Source: CAD feature listing. Evaluate the final solid. Frame: model axes, mm. A direction names the side the tool comes from. Give positions to 0.01 mm unless a question says otherwise; leave off trailing zeros. Write each loop counter-clockwise with the first axis right and the second up, starting at its lowest first coordinate (ties: lowest second). Pieces come first, ordered by that corner, then holes. Notation, with made-up numbers: (56.25, 19) - (61.25, 19) arc R11 cw to (61.25, 34) - close; hole circle Ø3 at (2.25, -19.75). An arc over 180 degrees is marked (long way). One line per question, with ' | ' between items. Start each with the question number.
(1) Section C-C, the plane x = -19.5. Return loops of the section in (y, z), plus the area to 3 significant figures.
(2) Draft query along Z for faces 4 (the flat face through (2.1, 0.7, -9)), 5 (the flat face through (-25.3, 5, -13.7)), 6 (the cylindrical face through (-26.58, 1.23, -17.6)), 7 (the cylindrical face through (26.58, 1.23, 17.6)). Return one class per face: +Z half, -Z half, draft (parallel to the pull), parting line (faces both ways), or undercut.
(3) Pin query (flat end, axial travel): pin 1 (1.9 mm diameter, centred on x = -24, z = 15, fed in from -Y); pin 2 (8 mm diameter, centred on x = -19, z = 6, fed in from +Y); pin 3 (1.7 mm diameter, centred on x = -0.5, z = 13, fed in from +Y). Return the tip coordinate at first contact, or that it passes through.
(4) Section B-B, the plane z = -7. Return loops of the section in (x, y), plus the area to 3 significant figures.
(5) Access query for faces 1 (the flat face through (4, 1, 0)), 2 (the flat face through (22.7, 5, -13.7)), 3 (the cylindrical face through (-24, 4, -18)). Directions: +Z, -Z, +X, -X, +Y, -Y. A direction counts if a zero-diameter tool reaches every point of the face in a straight line with its end or side. Return the directions, or none.
(6) Section A-A, the plane y = 4.1. Return loops of the section in (x, z), plus the area to 3 significant figures.
(7) Ray query, line 1 (Z direction, x = 24, y = 1.6); line 2 (X direction, y = 1.9, z = 15); line 3 (Z direction, x = -3, y = 2). Return the intervals inside material, ascending. Write a range as [from, to].
```python
from build123d import *

# Parameters (mm, degrees)
SKETCH_1_R           = 1.55
EXTRUDE_1_DEPTH      = 2.5
SKETCH_2_R           = 3
EXTRUDE_2_DEPTH      = 2.5
SKETCH_3_R           = 1.55
CUT_EXTRUDE_1_DEPTH  = 34.466573357
SKETCH_5_R           = 3.5
CUT_EXTRUDE_3_DEPTH  = 34.466573357
CUT_EXTRUDE_6_DEPTH  = 1.5
FILLET_4_R           = 0.5
CHAMFER_1_SIZE       = 2
CHAMFER_1_SIZE2      = 1
FILLET_5_R           = 1
CUT_EXTRUDE_7_DEPTH  = 34.466573357
SKETCH_20_W          = 5
SKETCH_20_H          = 18
CUT_EXTRUDE_10_DEPTH = 34.486179612
FILLET_9_R           = 1
SKETCH_23_R          = 1.05
CUT_EXTRUDE_11_DEPTH = 34.466573357
FILLET_10_R          = 1


with BuildPart() as part:
    # Sketch 1 → Extrude 1 (new body)
    with BuildSketch(Plane(origin=(0, 0, 0), x_dir=(1, 0, 0), z_dir=(0, 1, 0))):
        with BuildLine():
            Line((-27.4365, 0), (-27.4365, 15.5))
            ThreePointArc((-27.4365, 15.5), (-26.557820344, 17.621320344), (-24.4365, 18.5))
            Line((-24.4365, 18.5), (0, 18.5))
            Line((0, 18.5), (24.4365, 18.5))
            ThreePointArc((24.4365, 18.5), (26.557820344, 17.621320344), (27.4365, 15.5))
            Line((27.4365, 15.5), (27.4365, 0))
            Line((27.4365, 0), (27.4365, -15.5))
            ThreePointArc((27.4365, -15.5), (26.557820344, -17.621320344), (24.4365, -18.5))
            Line((24.4365, -18.5), (0, -18.5))
            Line((0, -18.5), (-24.4365, -18.5))
            ThreePointArc((-24.4365, -18.5), (-26.557820344, -17.621320344), (-27.4365, -15.5))
            Line((-27.4365, -15.5), (-27.4365, 0))
        make_face()
        with Locations(Location((-24, 15, 0), (0, 0, 270))):
            Circle(SKETCH_1_R, mode=Mode.SUBTRACT)
        with Locations(Location((24, 15, 0), (0, 0, 270))):
            Circle(SKETCH_1_R, mode=Mode.SUBTRACT)
        with Locations(Location((24, -15, 0), (0, 0, 90))):
            Circle(SKETCH_1_R, mode=Mode.SUBTRACT)
        with Locations(Location((-24, -15, 0), (0, 0, 90))):
            Circle(SKETCH_1_R, mode=Mode.SUBTRACT)
    extrude(amount=EXTRUDE_1_DEPTH)

    # Sketch 2 → Extrude 2 (add)
    with BuildSketch(Plane(origin=(0, 2.5, 0), x_dir=(1, 0, 0), z_dir=(0, 1, 0))):
        with Locations(Location((-24, 15, 0), (0, 0, 270))):
            Circle(SKETCH_2_R)
        with Locations(Location((24, 15, 0), (0, 0, 270))):
            Circle(SKETCH_2_R)
        with Locations(Location((-24, -15, 0), (0, 0, 270))):
            Circle(SKETCH_2_R)
        with Locations(Location((24, -15, 0), (0, 0, 270))):
            Circle(SKETCH_2_R)
    extrude(amount=EXTRUDE_2_DEPTH)

    # Sketch 3 → Cut-Extrude 1 (cut, through all)
    with BuildSketch(Plane.XZ):
        with Locations(Location((-24, 15, 0), (0, 0, 270))):
            Circle(SKETCH_3_R)
        with Locations(Location((24, 15, 0), (0, 0, 270))):
            Circle(SKETCH_3_R)
        with Locations(Location((-24, -15, 0), (0, 0, 270))):
            Circle(SKETCH_3_R)
        with Locations(Location((24, -15, 0), (0, 0, 270))):
            Circle(SKETCH_3_R)
    extrude(amount=-CUT_EXTRUDE_1_DEPTH, mode=Mode.SUBTRACT)

    # Sketch 5 → Cut-Extrude 3 (cut, through all)
    with BuildSketch(Plane.XZ):
        with Locations(Location((17, 0, 0), (0, 0, 270))):
            Circle(SKETCH_5_R)
    extrude(amount=-CUT_EXTRUDE_3_DEPTH, mode=Mode.SUBTRACT)

    # Sketch 9 → Cut-Extrude 6 (cut)
    with BuildSketch(Plane(origin=(0, 2.5, 0), x_dir=(1, 0, 0), z_dir=(0, 1, 0))):
        with BuildLine():
            Line((-2, -11.732050808), (2, -11.732050808))
            ThreePointArc((2, -11.732050808), (3.267949192, -13), (2, -14.267949192))
            Line((2, -14.267949192), (-2, -14.267949192))
            ThreePointArc((-2, -14.267949192), (-3.267949192, -13), (-2, -11.732050808))
        make_face()
    extrude(amount=-CUT_EXTRUDE_6_DEPTH, mode=Mode.SUBTRACT)

    # Fillet 4
    fillet_4_edges = [part.edges().sort_by_distance(p)[0] for p in [
        (0, 1, 14.267949192),
        (-3.267949192, 1, 13),
        (0, 1, 11.732050808),
        (3.267949192, 2.5, 13),
        (0, 2.5, 11.732050808),
        (-3.267949192, 2.5, 13),
        (0, 2.5, 14.267949192),
        (3.267949192, 1, 13),
    ]]
    fillet(fillet_4_edges, radius=FILLET_4_R)

    # Chamfer 1
    chamfer_1_edges = [part.edges().sort_by_distance(p)[0] for p in [
        (17, 0, 3.5),
    ]]
    chamfer_1_side = [part.faces().sort_by_distance(p)[0] for p in [
        (-0.334836292, 0, 0),
    ]]
    chamfer(chamfer_1_edges, length=CHAMFER_1_SIZE, length2=CHAMFER_1_SIZE2, reference=chamfer_1_side[0])

    # Fillet 5
    fillet_5_edges = [part.edges().sort_by_distance(p)[0] for p in [
        (17, 1, 3.5),
        (17, 0, 5.5),
    ]]
    fillet(fillet_5_edges, radius=FILLET_5_R)

    # Sketch 10 → Cut-Extrude 7 (cut, through all)
    with BuildSketch(Plane.XZ):
        Polygon((2.5, 0), (2.5, 9), (4, 9), (4, -9), (2.5, -9), align=None)
    extrude(amount=-CUT_EXTRUDE_7_DEPTH, mode=Mode.SUBTRACT)

    # Sketch 20 → Cut-Extrude 10 (cut, through all)
    with BuildSketch(Plane(origin=(-0.03944063, 0.086049296, 0), x_dir=(0.9090593428863095, 0.41666666666666674, 0), z_dir=(-0.4166666666666668, 0.9090593428863096, 0))):
        with Locations((0.293481691, 0)):
            Rectangle(SKETCH_20_W, SKETCH_20_H)
    extrude(amount=-CUT_EXTRUDE_10_DEPTH, mode=Mode.SUBTRACT)

    # Fillet 9
    fillet_9_edges = [part.edges().sort_by_distance(p)[0] for p in [
        (2.5, 2.5, 0),
        (-0.227178029, 0, 0),
    ]]
    fillet(fillet_9_edges, radius=FILLET_9_R)

    # Sketch 23 → Cut-Extrude 11 (cut, through all)
    with BuildSketch(Plane.XZ):
        with Locations(Location((-8.445435606, 5, 0), (0, 0, 270))):
            Circle(SKETCH_23_R)
        with Locations(Location((-8.445435606, -5, 0), (0, 0, 90))):
            Circle(SKETCH_23_R)
    extrude(amount=-CUT_EXTRUDE_11_DEPTH, mode=Mode.SUBTRACT)

    # Fillet 10
    fillet_10_edges = [part.edges().sort_by_distance(p)[0] for p in [
        (4, 1.25, 9),
        (4, 1.25, -9),
    ]]
    fillet(fillet_10_edges, radius=FILLET_10_R)


solid = part.part
```
Check sheet entries:
1) outline: (0, -18.5) - (2.5, -18.5) - (2.5, 18.5) - (0, 18.5) - close | area: 92.5 mm²
2) face 4: undercut | face 5: draft | face 6: -Z half | face 7: +Z half
3) pin 1: through | pin 2: y = 2.5 | pin 3: y = 1.01
4) outline: (-27.44, 0) - (-0.45, 0) arc R1 ccw to (-0.03, 0.09) - (2.5, 1.25) - (2.5, 1.5) arc R1 ccw to (1.5, 2.5) - (-27.44, 2.5) - close; (4, 0) - (27.44, 0) - (27.44, 2.5) - (4, 2.5) - close | area: 132 mm²
5) face 1: +Y, -Y | face 2: +Z, -Z, +X, -X, +Y | face 3: +Y
6) outline: circle Ø6 at (-24, -15); circle Ø6 at (-24, 15); circle Ø6 at (24, -15); circle Ø6 at (24, 15); hole circle Ø3.1 at (-24, -15); hole circle Ø3.1 at (-24, 15); hole circle Ø3.1 at (24, -15); hole circle Ø3.1 at (24, 15) | area: 82.9 mm²
7) line 1: [-18.5, -16.55], [-13.45, 13.45], [16.55, 18.5] | line 2: [-27.44, -25.55], [-22.45, 22.45], [25.55, 27.44] | line 3: [-18.5, 12.22], [13.78, 18.5]
